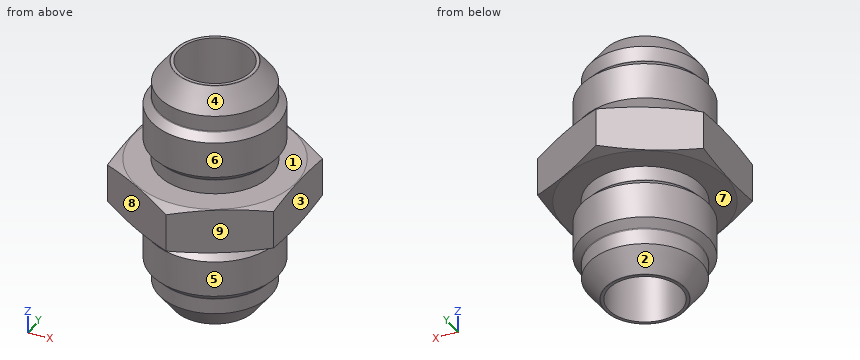
from build123d import *

# Parameters (mm, degrees)
CIRPATTERN1_COUNT   = 2
CIRPATTERN1_ANGLE   = 180
BOSS_EXTRUDE1_START = -4.8387
BOSS_EXTRUDE1_DEPTH = 9.6774
CIRPATTERN2_COUNT   = 2


with BuildPart() as part:
    # Sketch1 → Revolve1 (revolve)
    with BuildSketch(Plane(origin=(0, 0, 0), x_dir=(0, 0, -1), z_dir=(1, 0, 0))):
        with BuildLine():
            Line((-26.7843, 0), (0, 0))
            Line((0, 0), (0, 12.0015))
            Line((0, 12.0015), (-7.908489755, 12.0015))
            ThreePointArc((-7.908489755, 12.0015), (-8.005691347, 12.020834599), (-8.088094878, 12.075894878))
            Line((-8.088094878, 12.075894878), (-9.50595, 13.49375))
            Line((-9.50595, 13.49375), (-17.20215, 13.49375))
            Line((-17.20215, 13.49375), (-18.708905122, 11.986994878))
            ThreePointArc((-18.708905122, 11.986994878), (-18.791308653, 11.931934599), (-18.888510245, 11.9126))
            Line((-18.888510245, 11.9126), (-22.16644943, 11.9126))
            Line((-22.16644943, 11.9126), (-26.733730508, 8.470906846))
            ThreePointArc((-26.733730508, 8.470906846), (-26.770956664, 8.426147258), (-26.7843, 8.369480136))
            Line((-26.7843, 8.369480136), (-26.7843, 0))
        make_face()
    revolve(axis=Axis((0, 0, 19.812), (0, 0, -1)))


with BuildPart() as cirpattern1_1:
    # CirPattern1: pattern copy
    add(part.part.rotate(Axis((-10.4775, 0, 0), (1, 0, 0)), 1 * CIRPATTERN1_ANGLE / (CIRPATTERN1_COUNT - 1)))


with BuildPart() as part_1:
    add(part.part)

    add(cirpattern1_1.part)  # Boss-Extrude1 merges CirPattern1_1
    # Sketch4 → Boss-Extrude1 (add)
    with BuildSketch(Plane.XY.offset(BOSS_EXTRUDE1_START)):
        Polygon((0, 20.163958151), (-17.4625, 10.081979076), (-17.4625, -10.081979076), (0, -20.163958151), (17.4625, -10.081979076), (17.4625, 10.081979076), align=None)
    extrude(amount=BOSS_EXTRUDE1_DEPTH)

    # Sketch5 → Cut-Revolve1 (revolve, cut)
    with BuildSketch(Plane(origin=(0, 0, 0), x_dir=(0, 0, -1), z_dir=(1, 0, 0))):
        Polygon((-4.8387, 23.043216303), (4.8387, 23.043216303), (4.8387, 17.2847), (4.067205104, 20.163958151), (-4.067205104, 20.163958151), (-4.8387, 17.2847), align=None)
    revolve(axis=Axis((0, 0, 4.8387), (0, 0, -1)), mode=Mode.SUBTRACT)

    # Sketch6 → Cut-Revolve2 (revolve, cut)
    with BuildSketch(Plane(origin=(0, 0, 0), x_dir=(0, 0, -1), z_dir=(1, 0, 0))):
        with BuildLine():
            Line((-26.7843, 7.7343), (0, 7.7343))
            ThreePointArc((0, 7.7343), (5.468975978, 5.468975978), (7.7343, 0))
            Line((7.7343, 0), (-26.7843, 0))
            Line((-26.7843, 0), (-26.7843, 7.7343))
        make_face()
    cut_revolve2 = revolve(axis=Axis((0, 0, -7.7343), (0, 0, 1)), mode=Mode.SUBTRACT)

    # CirPattern2: Cut-Revolve2 ×2 about axis
    cirpattern2_axis = Axis((-10.4775, 0, 0), (1, 0, 0))
    for i in range(1, CIRPATTERN2_COUNT):
        add(cut_revolve2.rotate(cirpattern2_axis, i * 360 / CIRPATTERN2_COUNT), mode=Mode.SUBTRACT)


solid = part_1.part
Read the model definition and answer for the solid it produces. Units are mm, in the model's axes. Face numbers are marked on the shaded views. A direction names the side the tool comes from. Coordinates: 2 decimals unless noted, no trailing zeros. Loops run counter-clockwise (first coordinate to the right, second up) from the corner with the lowest first, then second, coordinate; pieces in that order, holes last. Notation, with made-up numbers: (82, 41) - (127, 41) arc R11 ccw to (127, 46) - close; hole circle Ø5 at (52, 87.5). An arc over 180 degrees is marked (long way). Answer in a Markdown table with one row per item.
Q1. The mould has two halves that part along Z. Classify the marked faces 1, 2, 3 and 4: pulls with the +Z half, pulls with the -Z half, needs draft (parallel to the pull), parting line crosses it, or undercut.
Here are the results:
| item | result |
|---|---|
| face 1 | undercut |
| face 2 | pulls with the -Z half |
| face 3 | needs draft |
| face 4 | pulls with the +Z half |
Q2. For the marked faces 5, 6, 7, 8 and 9, determine the directions among +Z, -Z, +X, -X, +Y, -Y from which every point of the face is accessible in a straight line to the end or side of a thin tool.
Here are the results:
| item | result |
|---|---|
| face 5 | -Z |
| face 6 | +Z |
| face 7 | none |
| face 8 | +Z, -Z, -X, -Y |
| face 9 | +Z, -Z, +X, -Y |
Q3. Given P1, Ø2, axis at y = 15.5, z = 16.5, coming from the +X side; P2, Ø6, axis at x = -12, y = 14, coming from the +Z side; P3, Ø3, axis at x = -5.5, z = -18, coming from the -Y side; P4, Ø10, axis at x = 1.5, z = -13.5, coming from the +Y side, each flat-ended and moving along its own axis, determine where each tip first touches the part or whether it passes through.
Here are the results:
| item | result |
|---|---|
| P1 | passes through |
| P2 | stops at z = 4.84 |
| P3 | stops at y = -12.81 |
| P4 | stops at y = 13.49 |
Q4. Straight lines are drawn through the part: line 1 along X through (y, z) = (0, 21); line 2 along X through (y, z) = (0, -13.5); line 3 along Z through (x, y) = (1, -17). For each, find the intervals that lie inside material, in ascending order. Write a range as [from, to].
Here are the results:
| item | result |
|---|---|
| line 1 | x = [-11.91, -7.73], [7.73, 11.91] |
| line 2 | x = [-13.49, -7.73], [7.73, 13.49] |
| line 3 | z = [-4.84, 4.84] |
Q5. Find section A-A on z = 5.5. Write down the section's boundary in (x, y), plus the area to 3 significant figures.
Here are the results:
| item | result |
|---|---|
| outline | circle Ø24 at (0, 0); hole circle Ø15.47 at (0, 0) |
| area | 265 mm^2 |
